Verification items for the finished model (mm, model axes). A direction names the side the tool comes from. Coordinates: 2 decimals unless noted, no trailing zeros. Loops run counter-clockwise (first coordinate to the right, second up) from the corner with the lowest first, then second, coordinate; pieces in that order, holes last. Notation, with made-up numbers: M 12.25,1 L 42.25,1 A21 ccw 42.25,22 Z; hole C -26,52 d5. An arc over 180 degrees is marked long. Write item = value, one per line. Start each with the question number.
```python
from build123d import *

# Parameters (mm, degrees)
BOSS_EXTRUDE1_DEPTH                                 = 12.7
CBORE_FOR_10_BINDING_HEAD_MACHINE_SCREW_D           = 5.1054
CBORE_FOR_10_BINDING_HEAD_MACHINE_SCREW_DEPTH       = 508
CBORE_FOR_10_BINDING_HEAD_MACHINE_SCREW_CBORE_D     = 11.1125
CBORE_FOR_10_BINDING_HEAD_MACHINE_SCREW_CBORE_DEPTH = 3.1242
CBORE_FOR_10_BINDING_HEAD_MACHINE_SCREW_TIP         = 1.533816902
SKETCH7_W                                           = 1.905
SKETCH7_H                                           = 44.45
CUT_EXTRUDE1_DEPTH                                  = 72.346425278
FILLET1_R                                           = 9.525


with BuildPart() as part:
    # Sketch1 → Boss-Extrude1 (new, symmetric)
    with BuildSketch(Plane(origin=(0, 0, 0), x_dir=(1, 0, 0), z_dir=(0, 1, 0))):
        with BuildLine():
            Line((-1.27, 10.975768811), (-1.27, 25.4))
            Line((-1.27, 25.4), (-20.32, 25.4))
            Line((-20.32, 25.4), (-20.32, -63.5))
            Line((-20.32, -63.5), (-1.27, -63.5))
            Line((-1.27, -63.5), (-1.27, -10.975768811))
            ThreePointArc((-1.27, -10.975768811), (-11.049, 0), (-1.27, 10.975768811))
        make_face()
    extrude(amount=BOSS_EXTRUDE1_DEPTH, both=True)

    # CBORE for #10 Binding Head Machine Screw1
    with Locations(Plane.ZY.offset(20.32)):
        with Locations((-19.05, 0), (34.29, 0), (53.34, 0)):
            CounterBoreHole(CBORE_FOR_10_BINDING_HEAD_MACHINE_SCREW_D / 2, CBORE_FOR_10_BINDING_HEAD_MACHINE_SCREW_CBORE_D / 2, CBORE_FOR_10_BINDING_HEAD_MACHINE_SCREW_CBORE_DEPTH, depth=CBORE_FOR_10_BINDING_HEAD_MACHINE_SCREW_DEPTH)
            with Locations((0, 0, -(CBORE_FOR_10_BINDING_HEAD_MACHINE_SCREW_DEPTH + CBORE_FOR_10_BINDING_HEAD_MACHINE_SCREW_TIP / 2))):  # 118° drill point
                Cone(0, CBORE_FOR_10_BINDING_HEAD_MACHINE_SCREW_D / 2, CBORE_FOR_10_BINDING_HEAD_MACHINE_SCREW_TIP, mode=Mode.SUBTRACT)

    # Sketch7 → Cut-Extrude1 (cut, through all)
    with BuildSketch(Plane(origin=(0, 12.7, 0), x_dir=(1, 0, 0), z_dir=(0, 1, 0))):
        with Locations((-2.2225, -41.275)):
            Rectangle(SKETCH7_W, SKETCH7_H)
    extrude(amount=-CUT_EXTRUDE1_DEPTH, mode=Mode.SUBTRACT)

    # Fillet1
    # the kernel refuses this fillet: 9.525 mm, written as the material it adds along each edge
    with BuildSketch(Plane(origin=(-3.175, 12.7, 19.05), x_dir=(1, 0, 0), z_dir=(0, -1, 0))) as fillet1_piece_1:
        with BuildLine():
            CenterArc((9.525, 5.715), FILLET1_R, 180, 36.869897646)
            Line((0, 5.715), (-0.1905, 5.715))
            Line((-0.1905, 5.715), (-0.1905, 0))
            Line((-0.1905, 0), (0, -0.1905))
            ThreePointArc((0, -0.1905), (0.9525, -0.1905), (1.7526, -0.1143))
            Line((1.7526, -0.1143), (1.905, 0))
        make_face()
    extrude(amount=25.4)


solid = part.part
```
Q1. Sectioned sample at B-B on y = 0. Count the separate pieces of the cut face and the enclosed holes in it, plus the area to 3 significant figures.
Q2. Scan lines: L1, parallel to Y at x = -3, z = -19; L2, parallel to Z at x = -19.5, y = -0.75; L3, parallel to X at y = -11.5, z = 34 (3 decimals). Record each from-to range of solid material in increasing order. Write a range as [from, to].
Q3. Sectioned sample at C-C on x = -16.25. Record the cut outline in (y, z).
Q4. Gauge pin test, flat ends, axial feed: pin 1 (3 mm diameter, centred on y = -2.5, z = -5.5, fed in from +X); pin 2 (8 mm diameter, centred on y = 0, z = 34.29, fed in from -X); pin 3 (3.5 mm diameter, centred on y = 0, z = -19.5, fed in from -X); pin 4 (7.5 mm diameter, centred on y = 2.5, z = 39.5, fed in from +X) (3 decimals). Record the tip position at first contact, or that the pin passes through.
Q5. Sectioned sample at D-D on y = 8.25. Record the cut outline in (x, z) (3 decimals).
Q6. Set-up check for faces 4 (the face through (-17.196, 1.31, -16.66)), 5 (the face through (-1.27, 0, 15)), 6 (the face through (-3.175, 0, 44)): record each of +Z, -Z, +X, -X, +Y, -Y from which the full face is reachable in a straight line by a thin tool's end or side.
Q7. Sectioned sample at A-A on z = 53.34. Record the cut outline in (x, y) (3 decimals), plus the area to 3 significant figures.
Q8. Mould release check, pull along Y, two halves, no side actions. Record for faces 1 (the face through (-10.09, 0.11, 36.84)), 2 (the face through (-13, -12.7, 20)), 3 (the face through (-20.32, 0, 18)): +Y half, -Y half, draft (parallel to the pull), parting line (faces both ways), or undercut.
Solutions:
q1.separate_pieces = 4
q1.enclosed_holes = 0
q1.area = 1,120 mm²
q2.L1 = [-12.7, -2.55], [2.55, 12.7]
q2.L2 = [-25.4, -24.56], [-13.54, 28.78], [39.8, 47.83], [58.85, 63.5]
q2.L3 = [-20.32, -3.175]
q3.outline = M -12.7,-25.4 L 12.7,-25.4 L 12.7,63.5 L -12.7,63.5 Z; hole C 0,-19.05 d5.11; hole C 0,34.29 d5.11; hole C 0,53.34 d5.11
q4.pin_1 = -8.55
q4.pin_2 = -17.2
q4.pin_3 = through
q4.pin_4 = -3.175
q5.outline = M -20.32,-25.4 L -1.27,-25.4 L -1.27,-10.976 A11.049 cw -1.27,10.976 L -1.27,19.05 A9.525 cw -3.175,24.765 L -3.175,63.5 L -20.32,63.5 Z
q6.face_4 = -X
q6.face_5 = +Z, -Z, +X, +Y, -Y
q6.face_6 = +Z, +X, +Y, -Y
q7.outline = M -20.32,-12.7 L -3.175,-12.7 L -3.175,-2.553 L -17.196,-2.553 L -17.196,-5.556 L -20.32,-5.556 Z; M -20.32,5.556 L -17.196,5.556 L -17.196,2.553 L -3.175,2.553 L -3.175,12.7 L -20.32,12.7 Z
q7.area = 329 mm²
q8.face_1 = undercut
q8.face_2 = -Y half
q8.face_3 = draft
